Model file for the job. Use its own axes, mm. A direction names the side the tool comes from. Coordinates: 2 decimals unless noted, no trailing zeros. Order: outer loops, then holes, each group sorted by start corner. A loop starts at its lowest first (then second) coordinate and runs counter-clockwise, first axis right, second up.
from build123d import *

# Parameters (mm, degrees)
CUT_EXTRUDE1_DEPTH = 10
CIRPATTERN1_COUNT  = 34
SKETCH4_R          = 2.3
CUT_EXTRUDE2_DEPTH = 13


with BuildPart() as part:
    # Sketch2 → Revolve1 (revolve)
    with BuildSketch(Plane(origin=(0, 0, 0), x_dir=(0, 0, -1), z_dir=(1, 0, 0)), mode=Mode.PRIVATE) as revolve1_sk:
        Polygon((-13, 5), (13, 5), (13, 30.23), (10, 30.23), (10, 26.1874), (0, 26.1874), (0, 28.2087), (0, 30.23), (-1.5, 30.23), (-3, 30.23), (-3, 15), (-13, 15), align=None)
    revolve(revolve1_sk.sketch.rotate(Axis((0, 0, 13), (0, 0, -1)), 90), axis=Axis((0, 0, 13), (0, 0, -1)))

    # Sketch3 → Cut-Extrude1 (cut)
    with BuildSketch(Plane.XY):
        with BuildLine():
            Line((-1.447918132, 25.537202459), (-1.45440268, 26.14698131))
            ThreePointArc((-1.45440268, 26.14698131), (0, 26.1874), (1.45440268, 26.14698131))
            Line((1.45440268, 26.14698131), (1.447918132, 25.537202459))
            ThreePointArc((1.447918132, 25.537202459), (0, 24.1046), (-1.447918132, 25.537202459))
        make_face()
    cut_extrude1 = extrude(amount=-CUT_EXTRUDE1_DEPTH, mode=Mode.SUBTRACT)

    # CirPattern1: Cut-Extrude1 ×34 about axis
    cirpattern1_axis = Axis((0, 0, 0), (0, 0, 1))
    for i in range(1, CIRPATTERN1_COUNT):
        add(cut_extrude1.rotate(cirpattern1_axis, i * 360 / CIRPATTERN1_COUNT), mode=Mode.SUBTRACT)

    # Sketch4 → Cut-Extrude2 (cut)
    with BuildSketch(Plane(origin=(0, 15, 0), x_dir=(1, 0, 0), z_dir=(0, 1, 0))):
        with Locations(Location((0, -8, 0), (0, 0, 270))):
            Circle(SKETCH4_R)
    extrude(amount=-CUT_EXTRUDE2_DEPTH, mode=Mode.SUBTRACT)


solid = part.part
Q1. Which spindle directions (+Z, -Z, +X, -X, +Y, -Y) get a long thin tool onto all of the face, cutting with end or side? Do faces 1 (the face through (22.272, -13.774, -4.93)), 2 (the face through (-19, -15, -5)), 3 (the face through (0.032, 24.105, -4.93)), 4 (the face through (-24.414, -9.473, -4.93)), 5 (the face through (-2.43, 26.074, -4.93)). Say none if no direction does.
Established:
face 1: +X, -Y
face 2: none
face 3: +Y
face 4: -X, -Y
face 5: -X, +Y
Q2. Probe line 1 (Z direction, x = -10, y = -28); line 2 (Z direction, x = 0, y = 12.5); line 3 (X direction, y = 8, z = 8). List the from-to ranges inside material, lowest first.
Established:
line 1: z = -13 to -10, 0 to 3
line 2: z = -13 to 5.7, 10.3 to 13
line 3: x = -12.69 to -2.3, 2.3 to 12.69
Q3. Mould opens along Z. For faces 6 (the face through (13.95, 26.82, 1.52)), 7 (the face through (26.187, 0.014, -4.93)) say: pulls with the +Z half, pulls with the -Z half, needs draft (parallel to the pull), parting line crosses it, or undercut.
Established:
face 6: needs draft
face 7: undercut
Q4. Cut at C-C, the plane z = 1. List the corners of the cut face in (x, y).
Established:
outline: circle Ø60.46 at (0, 0); hole circle Ø10 at (0, 0)
Q5. Cut at B-B, the plane x = 0. List the corners of the cut face in (y, z).
Established:
outline: (-30.23, -13) - (-5, -13) - (-5, 13) - (-15, 13) - (-15, 3) - (-30.23, 3) - (-30.23, 0) - (-24.1, 0) - (-24.1, -10) - (-30.23, -10) - close; (5, -13) - (30.23, -13) - (30.23, -10) - (24.1, -10) - (24.1, 0) - (30.23, 0) - (30.23, 3) - (15, 3) - (15, 5.7) - (5, 5.7) - close; (5, 10.3) - (15, 10.3) - (15, 13) - (5, 13) - close
Q6. Drop flat-ended pins along their axis: P1, Ø2, axis at x = -5.5, y = -20, coming from the +Z side; P2, Ø5, axis at x = -12, z = 1, coming from the -Y side; P3, Ø4, axis at x = 0, z = 8, coming from the +Y side; P4, Ø6, axis at x = 0, y = 0, coming from the -Z side. Give the stop position or say it passes through.
Established:
P1: stops at z = 3
P2: stops at y = -28.7
P3: stops at y = -4.58
P4: passes through
Q7. Cut at D-D, the plane x = 9.5. List the corners of the cut face in (y, z).
Established:
outline: (-28.7, -13) - (28.7, -13) - (28.7, -10) - (22.4, -10) - (22.4, 0) - (28.7, 0) - (28.7, 3) - (11.61, 3) - (11.61, 13) - (-11.61, 13) - (-11.61, 3) - (-28.7, 3) - (-28.7, 0) - (-22.4, 0) - (-22.4, -10) - (-28.7, -10) - close
Q8. Cut at A-A, the plane y = 0. List the corners of the cut face in (x, z), plus the area to 3 significant figures.
Established:
outline: (-30.23, -13) - (-5, -13) - (-5, 13) - (-15, 13) - (-15, 3) - (-30.23, 3) - (-30.23, 0) - (-26.19, 0) - (-26.19, -10) - (-30.23, -10) - close; (5, -13) - (30.23, -13) - (30.23, -10) - (26.19, -10) - (26.19, 0) - (30.23, 0) - (30.23, 3) - (15, 3) - (15, 13) - (5, 13) - close
area: 927 mm2
